Can you work these out from the model? Positions are in its coordinate system, mm. A direction names the side the tool comes from. Round coordinates to 2 decimals unless told otherwise and drop trailing zeros. Order: outer loops, then holes, each group sorted by start corner. A loop starts at its lowest first (then second) coordinate and runs counter-clockwise, first axis right, second up.
from build123d import *

# Parameters (mm, degrees)
SKETCH1_W           = 21
SKETCH1_H           = 12
BOSS_EXTRUDE1_DEPTH = 1.5
SKETCH2_R           = 2
CUT_EXTRUDE1_DEPTH  = 1.5
SKETCH3_W           = 8
SKETCH3_H           = 6
BOSS_EXTRUDE2_DEPTH = 3.5


with BuildPart() as part:
    # Sketch1 → Boss-Extrude1 (new body)
    with BuildSketch(Plane(origin=(0, 0, 0), x_dir=(1, 0, 0), z_dir=(0, 1, 0))):
        Rectangle(SKETCH1_W, SKETCH1_H)
    extrude(amount=BOSS_EXTRUDE1_DEPTH)

    # Sketch2 → Cut-Extrude1 (cut)
    with BuildSketch(Plane(origin=(0, 1.5, 0), x_dir=(1, 0, 0), z_dir=(0, 1, 0))):
        with Locations(Location((-7.5, 3, 0), (0, 0, 270))):
            Circle(SKETCH2_R)
        with Locations(Location((7.5, 3, 0), (0, 0, 270))):
            Circle(SKETCH2_R)
    extrude(amount=-CUT_EXTRUDE1_DEPTH, mode=Mode.SUBTRACT)

    # Sketch3 → Boss-Extrude2 (add)
    with BuildSketch(Plane(origin=(0, 1.5, 0), x_dir=(1, 0, 0), z_dir=(0, 1, 0))):
        with Locations((0, 3.5)):
            Rectangle(SKETCH3_W, SKETCH3_H)
    extrude(amount=BOSS_EXTRUDE2_DEPTH)


solid = part.part
(1) I'm going to push flat-ended pins straight in: pin 1 Ø4.5 at (x, z) = (7.5, -3) entering from -Y; pin 2 Ø4 at (x, z) = (7, -3) entering from +Y; pin 3 Ø3 at (x, z) = (-7.5, -3) entering from -Y; pin 4 Ø1.8 at (y, z) = (2.5, -4) entering from -X. Where does each tip first touch, or does it pass through?
(2) I want a section at A-A, the plane z = -3. List the corners of the cut face in (x, y) for me.
(3) On a 3-axis mill with a long thin cutter (end or side, diameter ignored), from which of +Z, -Z, +X, -X, +Y, -Y can I reach the whole of each face in a straight line? I mean faces 1 (the face through (0, 1, -6)), 2 (the face through (0, 3, -0.5)), 3 (the face through (9.483, 0.76, -3.26)). Say none if no direction works.
(4) I want a section at B-B, the plane x = 7.5. List the corners of the cut face in (y, z) for me.
(5) Please list where these lines run through material, in increasing order: probe 1 along X at (y, z) = (1.2, -3); probe 2 along Y at (x, z) = (-9, -0.25); probe 3 along Z at (x, y) = (3.75, 0.6).
(6) I want a section at C-C, the plane y = 0.7. List the corners of the cut face in (x, z) for me.
(7) If we mould it in two halves opening along X, with no side actions, what happens to faces 4 (the face through (4, 3, -3)), 5 (the face through (0, 3, -6.5)), 6 (the face through (-4, 3, -3)), 7 (the face through (-5.517, 0.76, -3.26))? For each: pulls with the +X half, pulls with the -X half, needs draft (parallel to the pull), parting line crosses it, or undercut.
(8) I want a section at D-D, the plane x = 1.5. List the corners of the cut face in (y, z) for me, plus the area to 3 significant figures.
Ans:
1. pin 1: stops at y = 0
1. pin 2: stops at y = 1.5
1. pin 3: passes through
1. pin 4: stops at x = -4
2. outline: (-10.5, 0) - (-9.5, 0) - (-9.5, 1.5) - (-10.5, 1.5) - close; (-5.5, 0) - (5.5, 0) - (5.5, 1.5) - (4, 1.5) - (4, 5) - (-4, 5) - (-4, 1.5) - (-5.5, 1.5) - close; (9.5, 0) - (10.5, 0) - (10.5, 1.5) - (9.5, 1.5) - close
3. face 1: -Z, +X, -X, -Y
3. face 2: +Z, +X, -X, +Y
3. face 3: +Y, -Y
4. outline: (0, -6) - (1.5, -6) - (1.5, -5) - (0, -5) - close; (0, -1) - (1.5, -1) - (1.5, 6) - (0, 6) - close
5. probe 1: x = -10.5 to -9.5, -5.5 to 5.5, 9.5 to 10.5
5. probe 2: y = 0 to 1.5
5. probe 3: z = -6 to 6
6. outline: (-10.5, -6) - (10.5, -6) - (10.5, 6) - (-10.5, 6) - close; hole circle Ø4 at (-7.5, -3); hole circle Ø4 at (7.5, -3)
7. face 4: pulls with the +X half
7. face 5: needs draft
7. face 6: pulls with the -X half
7. face 7: undercut
8. outline: (0, -6) - (1.5, -6) - (1.5, -6.5) - (5, -6.5) - (5, -0.5) - (1.5, -0.5) - (1.5, 6) - (0, 6) - close
8. area: 39.0 mm2
